Study the drawing (mm; zero at the part's minimum x, y, z) and answer. A direction names the side the tool comes from. Coordinates: 2 decimals unless noted, no trailing zeros. Order: outer loops, then holes, each group sorted by start corner. A loop starts at its lowest first (then second) coordinate and runs counter-clockwise, first axis right, second up. Notation, with made-up numbers: (36.5, 32) -> (94.5, 32) arc R20 ccw to (94.5, 45) -> close; hole circle Ø6 at (-32.75, 2). An arc over 180 degrees is marked (long way). Answer as CSV lines item,"result". Start each with the question number.
Item 1: Section A-A (y = 16) is taken. Write down the section's boundary in (x, z), then the cut area to 3 significant figures.
Item 2: Section C-C (x = 30) is taken. Write down the section's boundary in (y, z), then the cut area to 3 significant figures.
Item 3: Straight lines are drawn through the part: L1, parallel to Y at x = 5.08, z = 1.3 (3 decimals); L2, parallel to X at y = 7, z = 0.45; L3, parallel to Y at x = 27.5, z = 2.5. For each, find the intervals that lie inside material, in ascending order.
Item 4: Section B-B (x = 44.92) is taken. Write down the section's boundary in (y, z) (3 decimals), then the cut area to 3 significant figures.
Item 5: Which of the six approach directions +Z, -Z, +X, -X, +Y, -Y give full straight-line access (tool end or side, diameter ignored) to the marked faces 4 and 5?
Item 6: Each of these flat-tipped pins is pushed along its axis until it touches: pin 1 Ø2 at (y, z) = (17.5, 1.5) entering from -X; pin 2 Ø3 at (x, y) = (44.92, 7.045) entering from +Z. Where does it stop, or does it pass through?
Item 7: For a pull along X with two mould halves and no side action, classify the marked faces 1, 2 and 3 as pulls with the +X half, pulls with the -X half, needs draft (parallel to the pull), parting line crosses it, or undercut.
Item 8: Section D-D (z = 0.6) is taken. Write down the section's boundary in (x, y) (3 decimals), then the cut area to 3 significant figures.
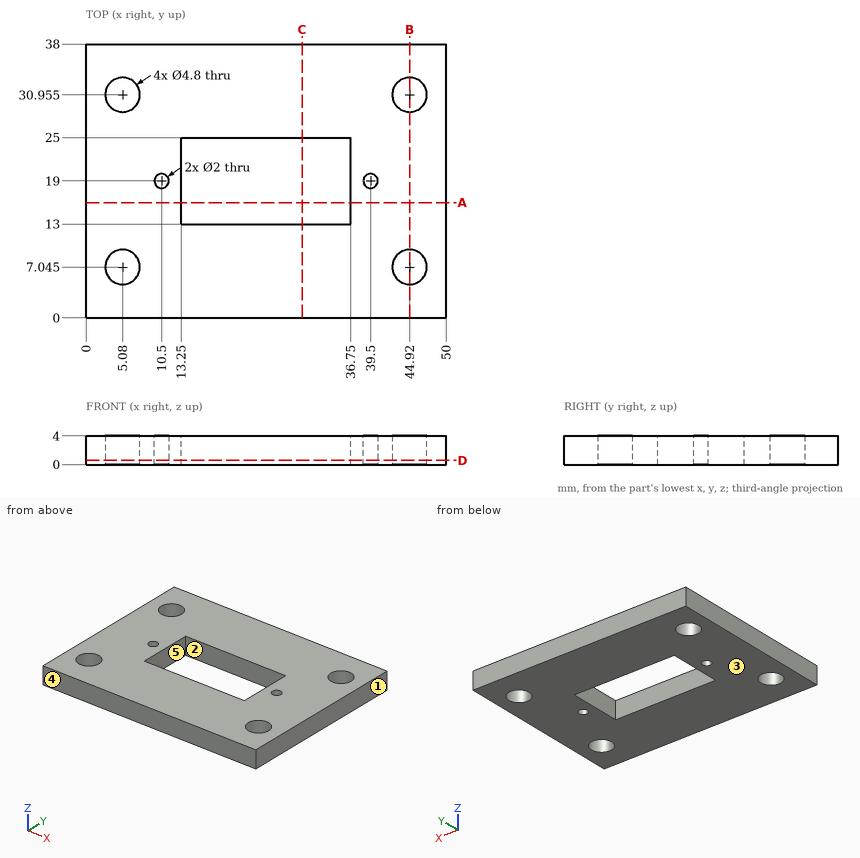
Checked values:
1,outline,"(0, 0) -> (13.25, 0) -> (13.25, 4) -> (0, 4) -> close; (36.75, 0) -> (50, 0) -> (50, 4) -> (36.75, 4) -> close"
1,area,"106 mm^2"
2,outline,"(0, 0) -> (13, 0) -> (13, 4) -> (0, 4) -> close; (25, 0) -> (38, 0) -> (38, 4) -> (25, 4) -> close"
2,area,"104 mm^2"
3,L1,"y = 0 to 4.645, 9.445 to 28.555, 33.355 to 38"
3,L2,"x = 0 to 2.68, 7.48 to 42.52, 47.32 to 50"
3,L3,"y = 0 to 13, 25 to 38"
4,outline,"(0, 0) -> (4.645, 0) -> (4.645, 4) -> (0, 4) -> close; (9.445, 0) -> (28.555, 0) -> (28.555, 4) -> (9.445, 4) -> close; (33.355, 0) -> (38, 0) -> (38, 4) -> (33.355, 4) -> close"
4,area,"114 mm^2"
5,face 4,"+Z, -Z, +X, -X, -Y"
5,face 5,"+Z, -Z"
6,pin 1,"stops at x = 0"
6,pin 2,"passes through"
7,face 1,"pulls with the +X half"
7,face 2,"undercut"
7,face 3,"needs draft"
8,outline,"(0, 0) -> (50, 0) -> (50, 38) -> (0, 38) -> close; hole circle Ø4.8 at (5.08, 7.045); hole circle Ø4.8 at (5.08, 30.955); hole circle Ø2 at (10.5, 19); hole (13.25, 13) -> (36.75, 13) -> (36.75, 25) -> (13.25, 25) -> close; hole circle Ø2 at (39.5, 19); hole circle Ø4.8 at (44.92, 7.045); hole circle Ø4.8 at (44.92, 30.955)"
8,area,"1,540 mm^2"
